Could you check a few things on this model? Use its own coordinates, in mm. Give positions to 0.01 mm unless a question says otherwise; leave off trailing zeros. Write each loop counter-clockwise with the first axis right and the second up, starting at its lowest first coordinate (ties: lowest second). Pieces come first, ordered by that corner, then holes. Notation, with made-up numbers: (5, -33.5) - (34, -33.5) arc R11 cw to (34, -21.5) - close; hole circle Ø2 at (-22, 33). An arc over 180 degrees is marked (long way). Answer in a Markdown table with one row per item.
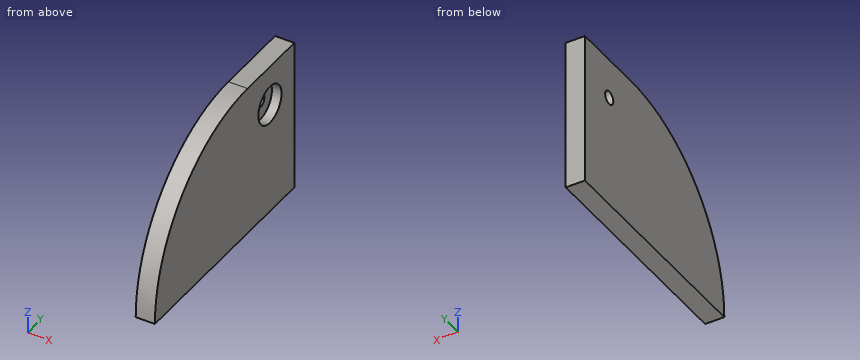
from build123d import *

# Parameters (mm, degrees)
PAD_DEPTH       = 5
SKETCH001_R     = 5
POCKET_DEPTH    = 2.5
SKETCH002_R     = 1.75
POCKET001_DEPTH = 5


with BuildPart() as part:
    # Sketch (on YZ_Plane of Origin) → Pad (new body)
    with BuildSketch(Plane.YZ):
        with BuildLine():
            Line((100, 15), (39.86189, 15))
            ThreePointArc((79.86189, 55), (51.577619, 43.284271), (39.86189, 15))
            Line((79.86189, 55), (100, 55))
            Line((100, 55), (100, 15))
        make_face()
    extrude(amount=PAD_DEPTH)

    # Sketch001 (on Face6 of Pad) → Pocket (cut)
    with BuildSketch(Plane.YZ.offset(5)):
        with Locations((89.5, 44.5)):
            Circle(SKETCH001_R)
    extrude(amount=-POCKET_DEPTH, mode=Mode.SUBTRACT)

    # Sketch002 (on Face8 of Pocket) → Pocket001 (cut)
    with BuildSketch(Plane.YZ.offset(2.5)):
        with Locations((89.5, 44.5)):
            Circle(SKETCH002_R)
    extrude(amount=-POCKET001_DEPTH, mode=Mode.SUBTRACT)


solid = part.part
1) Imagine slicing it at A-A (y = 89.5). List the corners of the cut face in (x, z) for me.
Check values:
| item | result |
|---|---|
| outline | (0, 15) - (5, 15) - (5, 39.5) - (2.5, 39.5) - (2.5, 42.75) - (0, 42.75) - close; (0, 46.25) - (2.5, 46.25) - (2.5, 49.5) - (5, 49.5) - (5, 55) - (0, 55) - close |
2) Imagine slicing it at C-C (x = 3.3). List the corners of the cut face in (y, z) for me, then the cut area to 3 significant figures.
Check values:
| item | result |
|---|---|
| outline | (39.86, 15) - (100, 15) - (100, 55) - (79.86, 55) arc R40 ccw to start; hole circle Ø10 at (89.5, 44.5) |
| area | 1,980 mm2 |
3) Imagine slicing it at D-D (z = 29). List the corners of the cut face in (x, y) for me, then the cut area to 3 significant figures.
Check values:
| item | result |
|---|---|
| outline | (0, 42.39) - (5, 42.39) - (5, 100) - (0, 100) - close |
| area | 288 mm2 |
4) If I drill on line 1 (Z direction, x = 3.9, y = 89.5); line 2 (Z direction, x = 1.95, y = 89.5); line 3 (Y direction, x = 2.9, z = 40), over which ranges is the centre line in solid material (lowest first)?
Check values:
| item | result |
|---|---|
| line 1 | z = 15 to 39.5, 49.5 to 55 |
| line 2 | z = 15 to 42.75, 46.25 to 55 |
| line 3 | y = 48.64 to 87.32, 91.68 to 100 |
5) Will these pins go through, and if not, where does the flat tip stop? P1, Ø6, axis at y = 89.5, z = 44.5, coming from the -X side; P2, Ø3, axis at y = 89.5, z = 44.5, coming from the +X side.
Check values:
| item | result |
|---|---|
| P1 | stops at x = 0 |
| P2 | passes through |
6) Imagine slicing it at B-B (z = 44.5). List the corners of the cut face in (x, y) for me.
Check values:
| item | result |
|---|---|
| outline | (0, 52.85) - (5, 52.85) - (5, 84.5) - (2.5, 84.5) - (2.5, 87.75) - (0, 87.75) - close; (0, 91.25) - (2.5, 91.25) - (2.5, 94.5) - (5, 94.5) - (5, 100) - (0, 100) - close |
